from build123d import *

# Parameters (mm, degrees)
SKETCH2_R           = 1.5
SKETCH2_R_2         = 3
BOSS_EXTRUDE1_DEPTH = 1.5
SKETCH3_R           = 1.25
F_45_DEGREES_DEPTH  = 170.629743854
SKETCH4_R           = 1.25
F_35_DEGRESS_DEPTH  = 170.629743854
FILLET1_R           = 5
FILLET2_R           = 5
FILLET3_R           = 5
FILLET4_R           = 5
FILLET5_R           = 5
FILLET6_R           = 5
FILLET7_R           = 5
FILLET8_R           = 5
FILLET10_R          = 5
FILLET11_R          = 5
FILLET12_R          = 5
FILLET13_R          = 5


with BuildPart() as part:
    # Sketch2 → Boss-Extrude1 (new body)
    with BuildSketch(Plane.XY):
        with BuildLine():
            Line((-79.195959493, 62.225396744), (-62.225396744, 79.195959493))
            ThreePointArc((-62.225396744, 79.195959493), (-44.806778225, 80.702789346), (-30, 90))
            Line((-30, 90), (30, 90))
            ThreePointArc((30, 90), (44.806778225, 80.702789346), (62.225396744, 79.195959493))
            Line((62.225396744, 79.195959493), (79.195959493, 62.225396744))
            ThreePointArc((79.195959493, 62.225396744), (57.477502656, 0), (79.195959493, -62.225396744))
            Line((79.195959493, -62.225396744), (62.225396744, -79.195959493))
            ThreePointArc((62.225396744, -79.195959493), (43.875108319, -77.923881554), (30, -90))
            Line((30, -90), (30, -135))
            ThreePointArc((30, -135), (25.606601718, -145.606601718), (15, -150))
            Line((15, -150), (-15, -150))
            ThreePointArc((-15, -150), (-25.606601718, -145.606601718), (-30, -135))
            Line((-30, -135), (-30, -90))
            ThreePointArc((-30, -90), (-43.875108319, -77.923881554), (-62.225396744, -79.195959493))
            Line((-62.225396744, -79.195959493), (-79.195959493, -62.225396744))
            ThreePointArc((-79.195959493, -62.225396744), (-57.477502656, 0), (-79.195959493, 62.225396744))
        make_face()
        with Locations((-37.5, 75)):
            Circle(SKETCH2_R, mode=Mode.SUBTRACT)
        with Locations((37.5, 75)):
            Circle(SKETCH2_R, mode=Mode.SUBTRACT)
        with Locations((37.5, -75)):
            Circle(SKETCH2_R, mode=Mode.SUBTRACT)
        with Locations((-37.5, -75)):
            Circle(SKETCH2_R, mode=Mode.SUBTRACT)
        with Locations((0, 84)):
            Circle(SKETCH2_R_2, mode=Mode.SUBTRACT)
        with BuildLine():
            Line((43, 5), (43, -5))
            ThreePointArc((43, -5), (40, -8), (37, -5))
            Line((37, -5), (37, 5))
            ThreePointArc((37, 5), (40, 8), (43, 5))
        make_face(mode=Mode.SUBTRACT)
        with BuildLine():
            Line((-43, 5), (-43, -5))
            ThreePointArc((-43, -5), (-40, -8), (-37, -5))
            Line((-37, -5), (-37, 5))
            ThreePointArc((-37, 5), (-40, 8), (-43, 5))
        make_face(mode=Mode.SUBTRACT)
    extrude(amount=BOSS_EXTRUDE1_DEPTH)

    # Sketch3 → 45 Degrees (cut, through all)
    with BuildSketch(Plane.XY.offset(1.5)):
        with Locations((-72.655221767, 60.280853096)):
            Circle(SKETCH3_R)
        with Locations((-58.513086143, 46.138717472)):
            Circle(SKETCH3_R)
        with Locations(Location((-60.280853096, 72.655221767, 0), (0, 0, 180))):
            Circle(SKETCH3_R)
        with Locations(Location((-46.138717472, 58.513086143, 0), (0, 0, 180))):
            Circle(SKETCH3_R)
        with Locations(Location((58.513086143, 46.138717472, 0), (0, 0, 180))):
            Circle(SKETCH3_R)
        with Locations(Location((72.655221767, 60.280853096, 0), (0, 0, 180))):
            Circle(SKETCH3_R)
        with Locations((60.280853096, 72.655221767)):
            Circle(SKETCH3_R)
        with Locations((46.138717472, 58.513086143)):
            Circle(SKETCH3_R)
        with Locations(Location((-58.513086143, -46.138717472, 0), (0, 0, 180))):
            Circle(SKETCH3_R)
        with Locations((-46.138717472, -58.513086143)):
            Circle(SKETCH3_R)
        with Locations((-60.280853096, -72.655221767)):
            Circle(SKETCH3_R)
        with Locations(Location((-72.655221767, -60.280853096, 0), (0, 0, 180))):
            Circle(SKETCH3_R)
        with Locations((58.513086143, -46.138717472)):
            Circle(SKETCH3_R)
        with Locations((72.655221767, -60.280853096)):
            Circle(SKETCH3_R)
        with Locations(Location((60.280853096, -72.655221767, 0), (0, 0, 180))):
            Circle(SKETCH3_R)
        with Locations(Location((46.138717472, -58.513086143, 0), (0, 0, 180))):
            Circle(SKETCH3_R)
    extrude(amount=-F_45_DEGREES_DEPTH, mode=Mode.SUBTRACT)

    # Sketch4 → 35 Degress (cut, through all)
    with BuildSketch(Plane.XY.offset(1.5)):
        with Locations((-70.197055442, 58.493417152)):
            Circle(SKETCH4_R)
        with Locations(Location((-60.280853096, 72.655221767, 0), (0, 0, 180))):
            Circle(SKETCH4_R)
        with Locations((60.280853096, 72.655221767)):
            Circle(SKETCH4_R)
        with Locations((-43.777344125, 61.357691434)):
            Circle(SKETCH4_R)
        with Locations((-53.814014556, 47.021888425)):
            Circle(SKETCH4_R)
        with Locations(Location((43.777344125, 61.357691434, 0), (0, 0, 180))):
            Circle(SKETCH4_R)
        with Locations(Location((53.814014556, 47.021888425, 0), (0, 0, 180))):
            Circle(SKETCH4_R)
        with Locations(Location((70.197055442, 58.493417152, 0), (0, 0, 180))):
            Circle(SKETCH4_R)
        with Locations(Location((60.280853096, -72.655221767, 0), (0, 0, 180))):
            Circle(SKETCH4_R)
        with Locations((70.197055442, -58.493417152)):
            Circle(SKETCH4_R)
        with Locations((43.777344125, -61.357691434)):
            Circle(SKETCH4_R)
        with Locations((53.814014556, -47.021888425)):
            Circle(SKETCH4_R)
        with Locations((-60.280853096, -72.655221767)):
            Circle(SKETCH4_R)
        with Locations(Location((-53.814014556, -47.021888425, 0), (0, 0, 180))):
            Circle(SKETCH4_R)
        with Locations(Location((-43.777344125, -61.357691434, 0), (0, 0, 180))):
            Circle(SKETCH4_R)
        with Locations(Location((-70.197055442, -58.493417152, 0), (0, 0, 180))):
            Circle(SKETCH4_R)
    extrude(amount=-F_35_DEGRESS_DEPTH, mode=Mode.SUBTRACT)

    # Fillet1
    fillet1_edges = [part.edges().sort_by_distance(p)[0] for p in [
        (-30, 90, 0.75),
    ]]
    fillet(fillet1_edges, radius=FILLET1_R)

    # Fillet2
    fillet2_edges = [part.edges().sort_by_distance(p)[0] for p in [
        (-79.195959493, 62.225396744, 0.75),
    ]]
    fillet(fillet2_edges, radius=FILLET2_R)

    # Fillet3
    fillet3_edges = [part.edges().sort_by_distance(p)[0] for p in [
        (-62.225396744, 79.195959493, 0.75),
    ]]
    fillet(fillet3_edges, radius=FILLET3_R)

    # Fillet4
    fillet4_edges = [part.edges().sort_by_distance(p)[0] for p in [
        (62.225396744, 79.195959493, 0.75),
    ]]
    fillet(fillet4_edges, radius=FILLET4_R)

    # Fillet5
    fillet5_edges = [part.edges().sort_by_distance(p)[0] for p in [
        (30, 90, 0.75),
    ]]
    fillet(fillet5_edges, radius=FILLET5_R)

    # Fillet6
    fillet6_edges = [part.edges().sort_by_distance(p)[0] for p in [
        (79.195959493, 62.225396744, 0.75),
    ]]
    fillet(fillet6_edges, radius=FILLET6_R)

    # Fillet7
    fillet7_edges = [part.edges().sort_by_distance(p)[0] for p in [
        (79.195959493, -62.225396744, 0.75),
    ]]
    fillet(fillet7_edges, radius=FILLET7_R)

    # Fillet8
    fillet8_edges = [part.edges().sort_by_distance(p)[0] for p in [
        (62.225396744, -79.195959493, 0.75),
    ]]
    fillet(fillet8_edges, radius=FILLET8_R)

    # Fillet10
    fillet10_edges = [part.edges().sort_by_distance(p)[0] for p in [
        (30, -90, 0.75),
    ]]
    fillet(fillet10_edges, radius=FILLET10_R)

    # Fillet11
    fillet11_edges = [part.edges().sort_by_distance(p)[0] for p in [
        (-30, -90, 0.75),
    ]]
    fillet(fillet11_edges, radius=FILLET11_R)

    # Fillet12
    fillet12_edges = [part.edges().sort_by_distance(p)[0] for p in [
        (-79.195959493, -62.225396744, 0.75),
    ]]
    fillet(fillet12_edges, radius=FILLET12_R)

    # Fillet13
    fillet13_edges = [part.edges().sort_by_distance(p)[0] for p in [
        (-62.225396744, -79.195959493, 0.75),
    ]]
    fillet(fillet13_edges, radius=FILLET13_R)


solid = part.part
Part model, mm, in its own coordinate system. Coordinates: 2 decimals unless noted, no trailing zeros. Order: outer loops, then holes, each group sorted by start corner. A loop starts at its lowest first (then second) coordinate and runs counter-clockwise, first axis right, second up.
(1) Slice it at B-B, the plane y = -122. Write the cut outline in (x, z).
Check sheet entries:
outline: (-30, 0) - (30, 0) - (30, 1.5) - (-30, 1.5) - close
(2) Pin check, flat tip, straight feed: pin 1 Ø6 at (x, y) = (-13.5, 65.5) entering from -Z. Stop position of the tip, or through.
Check sheet entries:
pin 1: stops at z = 0
(3) Slice it at C-C, the plane z = 0.6. State how many separate pieces and enclosed holes the cut face has, and give its area (3 significant figures).
Check sheet entries:
separate pieces: 1
enclosed holes: 35
area: 25,400 mm2
(4) Slice it at D-D, the plane y = 17. Write the cut outline in (x, z), and give its area (3 significant figures).
Check sheet entries:
outline: (-58.93, 0) - (58.93, 0) - (58.93, 1.5) - (-58.93, 1.5) - close
area: 177 mm2
(5) Pull direction X, two halves, no side cores. Call faces 1 (the face through (-42.88, -78.28, 0.74)), 2 (the face through (-70.11, 71.31, 0.74)), 3 (the face through (1, -2, 1.5)): pulls with the +X half, pulls with the -X half, needs draft (parallel to the pull), parting line crosses it, or undercut.
Check sheet entries:
face 1: undercut
face 2: pulls with the -X half
face 3: needs draft
(6) Probe L1, parallel to X at y = -2.5, z = 1.2; L2, parallel to X at y = -45, z = 0.3; L3, parallel to X at y = 28, z = 1.25. List the from-to ranges inside material, lowest first.
Check sheet entries:
L1: x = -57.51 to -43, -37 to 37, 43 to 57.51
L2: x = -68.17 to -59.03, -58 to 58, 59.03 to 68.17
L3: x = -61.48 to 61.48
(7) Slice it at A-A, the plane x = 0. Write the cut outline in (y, z), and give its area (3 significant figures).
Check sheet entries:
outline: (-150, 0) - (81, 0) - (81, 1.5) - (-150, 1.5) - close; (87, 0) - (90, 0) - (90, 1.5) - (87, 1.5) - close
area: 351 mm2
